```python
from build123d import *

# Parameters (mm, degrees)
SKETCH1_R           = 10
BOSS_EXTRUDE1_DEPTH = 15
SKETCH2_R           = 13
BOSS_EXTRUDE2_DEPTH = 3


# Read off the part's stored shape, not the designer's step: G3/8 Straight Pipe Tapped Thread Stud1
with BuildPart() as part:
    # Sketch1 → Boss-Extrude1 (new body)
    with BuildSketch(Plane(origin=(0, 0, 0), x_dir=(0, 0, -1), z_dir=(1, 0, 0))):
        Circle(SKETCH1_R)
    extrude(amount=BOSS_EXTRUDE1_DEPTH)

    # Sketch2 → Boss-Extrude2 (add)
    with BuildSketch(Plane.ZY):
        Circle(SKETCH2_R)
    extrude(amount=BOSS_EXTRUDE2_DEPTH)

    # G3/8 Straight Pipe Tapped Thread Stud1 o → G3/8 Straight Pipe Tapped Thread Stud1 (revolve, cut)
    with BuildSketch(Plane.YX):
        Polygon((10, 15), (7.475, 15), (8.331, 14.144), (8.331, 0), (10, 0), align=None)
    revolve(axis=Axis((0, 0, 0), (1, 0, 0)), mode=Mode.SUBTRACT)


solid = part.part
```
The listing builds one solid part. Answer for the finished solid, in the listing's coordinates (mm). A direction names the side the tool comes from. Coordinates: 2 decimals unless noted, no trailing zeros. Write each loop counter-clockwise with the first axis right and the second up, starting at its lowest first coordinate (ties: lowest second). Pieces come first, ordered by that corner, then holes.
Q1. Given P1, Ø5, axis at x = 8.5, z = 7, coming from the -Y side; P2, Ø6, axis at x = 10.5, z = -6.5, coming from the +Y side; P3, Ø1.5, axis at x = 6, y = -7.5, coming from the -Z side, each flat-ended and moving along its own axis, determine where each tip first touches the part or whether it passes through.
Returned:
P1: stops at y = -7.01
P2: stops at y = 7.56
P3: stops at z = -4.88
Q2. Which of the six approach directions +Z, -Z, +X, -X, +Y, -Y give full straight-line access (tool end or side, diameter ignored) to faces 1 (the flat face through (15, 0, 0)), 2 (the cylindrical face through (6.97, -1.81, -8.13))?
Returned:
face 1: +Z, -Z, +X, +Y, -Y
face 2: +X
Q3. Section D-D, the plane z = 11 is taken. Write down the section's boundary in (x, y), then the cut area to 3 significant figures.
Returned:
outline: (-3, -6.93) - (0, -6.93) - (0, 6.93) - (-3, 6.93) - close
area: 41.6 mm2
Q4. Section C-C, the plane x = 10 is taken. Write down the section's boundary in (y, z).
Returned:
outline: circle Ø16.66 at (0, 0)
Q5. Section A-A, the plane y = 0 is taken. Write down the section's boundary in (x, z) (3 decimals).
Returned:
outline: (-3, -13) - (0, -13) - (0, -8.331) - (14.144, -8.331) - (15, -7.475) - (15, 7.475) - (14.144, 8.331) - (0, 8.331) - (0, 13) - (-3, 13) - close
Q6. Find the intervals of material crossed by line 1 along X through (y, z) = (8.5, -3); line 2 along X through (y, z) = (-1.75, 7.5); line 3 along Y through (x, z) = (8, -7.25), in increasing order.
Returned:
line 1: x = -3 to 0
line 2: x = -3 to 14.77
line 3: y = -4.1 to 4.1
